Answer from the drawing. Dimensions are ordinates in mm from the lowest x, y and z of the part. A direction names the side the tool comes from. Round coordinates to 2 decimals unless told otherwise and drop trailing zeros. Loops run counter-clockwise (first coordinate to the right, second up) from the corner with the lowest first, then second, coordinate; pieces in that order, holes last. Notation, with made-up numbers: M 19,10 L 57,10 A29 cw 57,44 Z; hole C 36,12.5 d5. An arc over 180 degrees is marked long. Answer as a JSON object with one key per item and string values.
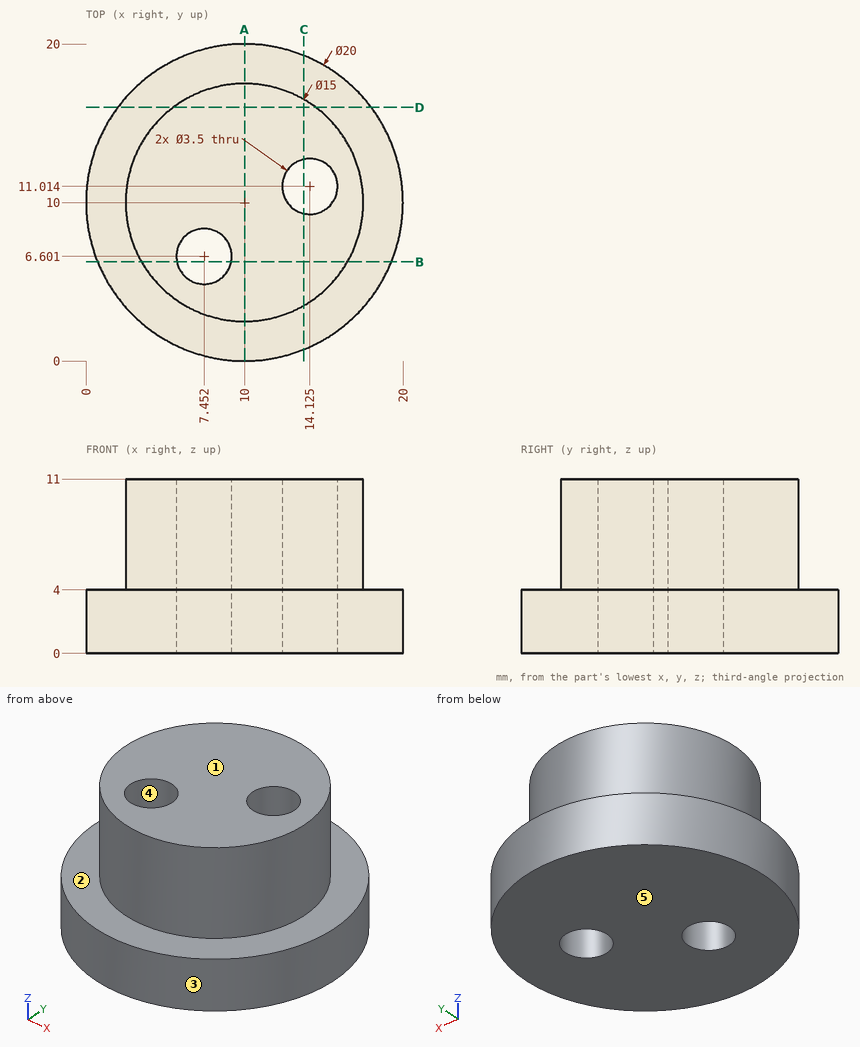
Item 1: Determine the mould class of the marked faces 3, 4 and 5 for opening direction Y: released by +Y, released by -Y, zero draft, split by the parting line, or undercut.
Values follow:
{"face 3": "split by the parting line", "face 4": "undercut", "face 5": "zero draft"}
Item 2: The part is cut by section C-C (x = 13.75). Give the vertices of the cut face in (y, z) (1 decimal).
Values follow:
{"outline": "M 0.7,0 L 9.3,0 L 9.3,11 L 3.5,11 L 3.5,4 L 0.7,4 Z; M 12.7,0 L 19.3,0 L 19.3,4 L 16.5,4 L 16.5,11 L 12.7,11 Z"}
Item 3: The part is cut by section B-B (y = 6.25). Give the vertices of the cut face in (x, z) (1 decimal), then the cut area to 3 significant figures.
Values follow:
{"outline": "M 0.7,0 L 5.7,0 L 5.7,11 L 3.5,11 L 3.5,4 L 0.7,4 Z; M 9.2,0 L 19.3,0 L 19.3,4 L 16.5,4 L 16.5,11 L 9.2,11 Z", "area": "127 mm^2"}
Item 4: Which of the six approach directions +Z, -Z, +X, -X, +Y, -Y give full straight-line access (tool end or side, diameter ignored) to the marked faces 1 and 2?
Values follow:
{"face 1": "+Z, +X, -X, +Y, -Y", "face 2": "+Z"}
Item 5: Flat-ended cylindrical pins translate along their axes: P1, Ø6, axis at x = 4, y = 2.5, coming from the -Z side; P2, Ø1.5, axis at y = 13.5, z = 2.5, coming from the -X side (1 decimal); P3, Ø2, axis at x = 4.5, z = 1.5, coming from the +Y side; P4, Ø3, axis at y = 9.5, z = 8, coming from the -X side. Find the tip coordinate at first contact, or state that the pin passes through.
Values follow:
{"P1": "z = 0", "P2": "x = 0.4", "P3": "y = 18.93", "P4": "x = 2.5"}
Item 6: The part is cut by section D-D (y = 16). Give the vertices of the cut face in (x, z), then the cut area to 3 significant figures.
Values follow:
{"outline": "M 2,0 L 18,0 L 18,4 L 14.5,4 L 14.5,11 L 5.5,11 L 5.5,4 L 2,4 Z", "area": "127 mm^2"}
Item 7: Straight lines are drawn through the part: line 1 (Z direction, x = 1.75, y = 13.75); line 2 (X direction, y = 5.5, z = 4.5); line 3 (Y direction, x = 14, z = 5) (1 decimal). For each, find the intervals that lie inside material, in ascending order.
Values follow:
{"line 1": "0 to 4", "line 2": "4 to 6.09, 8.81 to 16", "line 3": "3.7 to 9.3, 12.8 to 16.3"}
Item 8: The part is cut by section A-A (x = 10). Give the vertices of the cut face in (y, z), then the cut area to 3 significant figures.
Values follow:
{"outline": "M 0,0 L 20,0 L 20,4 L 17.5,4 L 17.5,11 L 2.5,11 L 2.5,4 L 0,4 Z", "area": "185 mm^2"}
